```python
from build123d import *

# Parameters (mm, degrees)
SALIENTE_EXTRUIR1_DEPTH          = 3.1
SALIENTE_EXTRUIR2_DEPTH          = 3
SALIENTE_EXTRUIR3_DEPTH          = 3
TALADRO_DE_MARGEN_PARA_M41_D     = 4.5
TALADRO_DE_MARGEN_PARA_M41_DEPTH = 8.2
TALADRO_DE_MARGEN_PARA_M41_TIP   = 1.351936393
CROQUIS10_W                      = 11.5
CROQUIS10_H                      = 11.5
SALIENTE_EXTRUIR4_DEPTH          = 87
SALIENTE_EXTRUIR5_DEPTH          = 12
CROQUIS14_R                      = 2
CORTAR_EXTRUIR1_DEPTH            = 6
CHAFL_N1_SIZE                    = 0.3
TALADRO_DE_MARGEN_PARA_M61_D     = 6.6
TALADRO_DE_MARGEN_PARA_M61_DEPTH = 8.2
TALADRO_DE_MARGEN_PARA_M61_TIP   = 1.982840043
CORTAR_EXTRUIR3_DEPTH            = 12
REDONDEO1_R                      = 2.5
CROQUIS19_R                      = 6.15
SALIENTE_EXTRUIR6_DEPTH          = 12
CROQUIS20_R                      = 2.85
CORTAR_EXTRUIR4_DEPTH            = 8.2
CHAFL_N2_SIZE                    = 0.5


with BuildPart() as part:
    # Croquis4 → Saliente-Extruir1 (new body)
    with BuildSketch(Plane(origin=(0, 0, 6.1), x_dir=(-1, 0, 0), z_dir=(0, 0, -1))):
        with BuildLine():
            Line((-120.1, -80.5), (-120.1, 80.5))
            ThreePointArc((-120.1, 80.5), (-121.271572875, 83.328427125), (-124.1, 84.5))
            Line((-124.1, 84.5), (-329.1, 84.5))
            ThreePointArc((-329.1, 84.5), (-331.928427125, 83.328427125), (-333.1, 80.5))
            Line((-333.1, 80.5), (-333.1, -80.5))
            ThreePointArc((-333.1, -80.5), (-331.928427125, -83.328427125), (-329.1, -84.5))
            Line((-329.1, -84.5), (-124.1, -84.5))
            ThreePointArc((-124.1, -84.5), (-121.271572875, -83.328427125), (-120.1, -80.5))
        make_face()
    extrude(amount=SALIENTE_EXTRUIR1_DEPTH)



with BuildPart() as body_2:
    # Croquis5 → Saliente-Extruir2 (new body)
    with BuildSketch(Plane(origin=(0, 0, 3), x_dir=(-1, 0, 0), z_dir=(0, 0, -1))):
        with BuildLine():
            Line((-326.1, 59), (-326.1, -59))
            Line((-326.1, -59), (-326.1, -75))
            ThreePointArc((-326.1, -75), (-325.367766953, -76.767766953), (-323.6, -77.5))
            Line((-323.6, -77.5), (-129.6, -77.5))
            ThreePointArc((-129.6, -77.5), (-127.832233047, -76.767766953), (-127.1, -75))
            Line((-127.1, -75), (-127.1, 75))
            ThreePointArc((-127.1, 75), (-127.832233047, 76.767766953), (-129.6, 77.5))
            Line((-129.6, 77.5), (-323.6, 77.5))
            ThreePointArc((-323.6, 77.5), (-325.367766953, 76.767766953), (-326.1, 75))
            Line((-326.1, 75), (-326.1, 59))
        make_face()
        with BuildLine():
            Line((-324.1, 59), (-324.1, -59))
            Line((-324.1, -59), (-324.1, -75))
            ThreePointArc((-324.1, -75), (-323.953553391, -75.353553391), (-323.6, -75.5))
            Line((-323.6, -75.5), (-129.6, -75.5))
            ThreePointArc((-129.6, -75.5), (-129.246446609, -75.353553391), (-129.1, -75))
            Line((-129.1, -75), (-129.1, 75))
            ThreePointArc((-129.1, 75), (-129.246446609, 75.353553391), (-129.6, 75.5))
            Line((-129.6, 75.5), (-323.6, 75.5))
            ThreePointArc((-323.6, 75.5), (-323.953553391, 75.353553391), (-324.1, 75))
            Line((-324.1, 75), (-324.1, 59))
        make_face(mode=Mode.SUBTRACT)
    extrude(amount=SALIENTE_EXTRUIR2_DEPTH)


with BuildPart() as part_1:
    add(part.part)

    add(body_2.part)  # Saliente-Extruir3 merges body 2
    # Croquis6 → Saliente-Extruir3 (add)
    with BuildSketch(Plane(origin=(0, 0, 3), x_dir=(-1, 0, 0), z_dir=(0, 0, -1))):
        with BuildLine():
            Line((-120.1, -80.5), (-120.1, 80.5))
            ThreePointArc((-120.1, 80.5), (-121.271572875, 83.328427125), (-124.1, 84.5))
            Line((-124.1, 84.5), (-329.1, 84.5))
            ThreePointArc((-329.1, 84.5), (-331.928427125, 83.328427125), (-333.1, 80.5))
            Line((-333.1, 80.5), (-333.1, -80.5))
            ThreePointArc((-333.1, -80.5), (-331.928427125, -83.328427125), (-329.1, -84.5))
            Line((-329.1, -84.5), (-124.1, -84.5))
            ThreePointArc((-124.1, -84.5), (-121.271572875, -83.328427125), (-120.1, -80.5))
        make_face()
        with BuildLine():
            Line((-122.1, -80.5), (-122.1, 80.5))
            ThreePointArc((-122.1, 80.5), (-122.685786438, 81.914213562), (-124.1, 82.5))
            Line((-124.1, 82.5), (-329.1, 82.5))
            ThreePointArc((-329.1, 82.5), (-330.514213562, 81.914213562), (-331.1, 80.5))
            Line((-331.1, 80.5), (-331.1, -80.5))
            ThreePointArc((-331.1, -80.5), (-330.514213562, -81.914213562), (-329.1, -82.5))
            Line((-329.1, -82.5), (-124.1, -82.5))
            ThreePointArc((-124.1, -82.5), (-122.685786438, -81.914213562), (-122.1, -80.5))
        make_face(mode=Mode.SUBTRACT)
    extrude(amount=SALIENTE_EXTRUIR3_DEPTH)

    # Taladro de margen para M41
    with Locations(Plane.XY.offset(6.1)):
        with Locations((151.35, 20.5), (206.45, 20.5), (206.45, -20.5), (151.35, -20.5)):
            Hole(TALADRO_DE_MARGEN_PARA_M41_D / 2, depth=TALADRO_DE_MARGEN_PARA_M41_DEPTH)
            with Locations((0, 0, -(TALADRO_DE_MARGEN_PARA_M41_DEPTH + TALADRO_DE_MARGEN_PARA_M41_TIP / 2))):  # 118° drill point
                Cone(0, TALADRO_DE_MARGEN_PARA_M41_D / 2, TALADRO_DE_MARGEN_PARA_M41_TIP, mode=Mode.SUBTRACT)

    # Croquis10 → Saliente-Extruir4 (add)
    with BuildSketch(Plane(origin=(0, 0, 3), x_dir=(-1, 0, 0), z_dir=(0, 0, -1))):
        with Locations((-132.85, 71.75)):
            Rectangle(CROQUIS10_W, CROQUIS10_H)
        with Locations((-132.85, -71.75)):
            Rectangle(CROQUIS10_W, CROQUIS10_H)
        with Locations((-320.35, -71.75)):
            Rectangle(CROQUIS10_W, CROQUIS10_H)
        with Locations((-320.35, 71.75)):
            Rectangle(CROQUIS10_W, CROQUIS10_H)
    extrude(amount=SALIENTE_EXTRUIR4_DEPTH)

    # Croquis13 → Saliente-Extruir5 (add)
    with BuildSketch(Plane(origin=(0, 0, 3), x_dir=(-1, 0, 0), z_dir=(0, 0, -1))):
        Polygon((-213.1, -55), (-323.1, -55), (-323.1, 55), (-213.1, 55), (-213.1, 21.5), (-209.1, 21.5), (-209.1, 59), (-326.1, 59), (-326.1, -59), (-209.1, -59), (-209.1, -21.5), (-213.1, -21.5), align=None)
    extrude(amount=SALIENTE_EXTRUIR5_DEPTH)

    # Croquis14 → Cortar-Extruir1 (cut)
    with BuildSketch(Plane(origin=(0, 0, -84), x_dir=(-1, 0, 0), z_dir=(0, 0, -1))):
        with Locations((-132.85, -71.75)):
            Circle(CROQUIS14_R)
        with Locations((-132.85, 71.75)):
            Circle(CROQUIS14_R)
        with Locations((-320.35, 71.75)):
            Circle(CROQUIS14_R)
        with Locations((-320.35, -71.75)):
            Circle(CROQUIS14_R)
    extrude(amount=-CORTAR_EXTRUIR1_DEPTH, mode=Mode.SUBTRACT)

    # Chaflán1
    chafl_n1_edges = [part_1.edges().sort_by_distance(p)[0] for p in [
        (322.35, -71.75, -84),
        (322.35, 71.75, -84),
        (134.85, 71.75, -84),
        (134.85, -71.75, -84),
    ]]
    chamfer(chafl_n1_edges, length=CHAFL_N1_SIZE)

    # Taladro de margen para M61
    with Locations(Plane.XY.offset(6.1)):
        with Locations((229.4, 69.675), (229.4, -69.675)):
            Hole(TALADRO_DE_MARGEN_PARA_M61_D / 2, depth=TALADRO_DE_MARGEN_PARA_M61_DEPTH)
            with Locations((0, 0, -(TALADRO_DE_MARGEN_PARA_M61_DEPTH + TALADRO_DE_MARGEN_PARA_M61_TIP / 2))):  # 118° drill point
                Cone(0, TALADRO_DE_MARGEN_PARA_M61_D / 2, TALADRO_DE_MARGEN_PARA_M61_TIP, mode=Mode.SUBTRACT)

    # Croquis18 → Cortar-Extruir3 (cut)
    with BuildSketch(Plane(origin=(0, 0, -9), x_dir=(-1, 0, 0), z_dir=(0, 0, -1))):
        Polygon((-212.6, 21.5), (-212.6, 55.5), (-323.6, 55.5), (-323.6, -55.5), (-212.6, -55.5), (-212.6, -21.5), (-213.1, -21.5), (-213.1, -55), (-323.1, -55), (-323.1, 55), (-213.1, 55), (-213.1, 21.5), align=None)
    extrude(amount=-CORTAR_EXTRUIR3_DEPTH, mode=Mode.SUBTRACT)

    # Redondeo1
    redondeo1_edges = [part_1.edges().sort_by_distance(p)[0] for p in [
        (127.1, 77.5, -40.5),
        (127.1, -77.5, -40.5),
        (326.1, -77.5, -40.5),
        (326.1, 77.5, -40.5),
    ]]
    fillet(redondeo1_edges, radius=REDONDEO1_R)

    # Croquis19 → Saliente-Extruir6 (add)
    with BuildSketch(Plane(origin=(0, 0, 3), x_dir=(-1, 0, 0), z_dir=(0, 0, -1))):
        with Locations(Location((-151.35, -20.5, 0), (0, 0, 270))):
            Circle(CROQUIS19_R)
        with Locations(Location((-151.35, 20.5, 0), (0, 0, 270))):
            Circle(CROQUIS19_R)
        with Locations((-206.45, 20.5)):
            Circle(CROQUIS19_R)
        with Locations((-206.45, -20.5)):
            Circle(CROQUIS19_R)
    extrude(amount=SALIENTE_EXTRUIR6_DEPTH)

    # Croquis20 → Cortar-Extruir4 (cut)
    with BuildSketch(Plane.XY.offset(6.1)):
        with Locations((151.35, -20.5)):
            Circle(CROQUIS20_R)
        with Locations((206.45, -20.5)):
            Circle(CROQUIS20_R)
        with Locations((206.45, 20.5)):
            Circle(CROQUIS20_R)
        with Locations((151.35, 20.5)):
            Circle(CROQUIS20_R)
    extrude(amount=-CORTAR_EXTRUIR4_DEPTH, mode=Mode.SUBTRACT)

    # Chaflán2
    chafl_n2_edges = [part_1.edges().sort_by_distance(p)[0] for p in [
        (148.5, 20.5, 6.1),
        (203.6, 20.5, 6.1),
        (203.6, -20.5, 6.1),
        (148.5, -20.5, 6.1),
    ]]
    chamfer(chafl_n2_edges, length=CHAFL_N2_SIZE)


solid = part_1.part
```
CAD build for the part. Positions are in the model's coordinates, mm. A direction names the side the tool comes from. Give positions to 0.01 mm unless a question says otherwise; leave off trailing zeros. Loops run counter-clockwise (first coordinate to the right, second up) from the corner with the lowest first, then second, coordinate; pieces in that order, holes last. Notation, with made-up numbers: (61, -31) - (110, -31) arc R17 ccw to (110, -9) - close; hole circle Ø5 at (47.25, 39). An arc over 180 degrees is marked (long way). Put each result on its own line as item: value.
Q1. Slice it at B-B (x = 166). Give the cut face in (y, z), plus the area to 3 significant figures.
Filled in:
outline: (-84.5, 0) - (-82.5, 0) - (-82.5, 3) - (-77.5, 3) - (-77.5, 0) - (-75.5, 0) - (-75.5, 3) - (75.5, 3) - (75.5, 0) - (77.5, 0) - (77.5, 3) - (82.5, 3) - (82.5, 0) - (84.5, 0) - (84.5, 6.1) - (-84.5, 6.1) - close
area: 548 mm²
Q2. Mould opens along Y. For faces 4 (the face through (267, 59, -3)), 5 (the face through (228, 1, 6.1)), 6 (the face through (228, -84.5, 3)), 7 (the face through (206, 21, -2.1)) say: pulls with the +Y half, pulls with the -Y half, needs draft (parallel to the pull), parting line crosses it, or undercut.
Filled in:
face 4: undercut
face 5: needs draft
face 6: pulls with the -Y half
face 7: undercut
Q3. Slice it at A-A (z = -33). Give the cut face in (x, y).
Filled in:
outline: (127.1, -75) arc R2.5 ccw to (129.6, -77.5) - (138.6, -77.5) - (138.6, -66) - (127.1, -66) - close; (127.1, 66) - (138.6, 66) - (138.6, 77.5) - (129.6, 77.5) arc R2.5 ccw to (127.1, 75) - close; (314.6, -77.5) - (323.6, -77.5) arc R2.5 ccw to (326.1, -75) - (326.1, -66) - (314.6, -66) - close; (314.6, 66) - (326.1, 66) - (326.1, 75) arc R2.5 ccw to (323.6, 77.5) - (314.6, 77.5) - close
Q4. Flat gauge pins, fed straight in: pin 1 (8 mm diameter, centred on y = 6.5, z = -9.5, fed in from +X); pin 2 (9 mm diameter, centred on x = 133, z = -62, fed in from -Y); pin 3 (3 mm diameter, centred on x = 206, y = 21, fed in from +Z); pin 4 (6 mm diameter, centred on y = 62, z = -53.5, fed in from -X). Where does each tip first touch, or does it go through?
Filled in:
pin 1: stops at x = 326.1
pin 2: stops at y = -77.5
pin 3: stops at z = -2.1
pin 4: passes through
Q5. Probe line 1 along Y through (x, z) = (320, -81); line 2 along Y through (x, z) = (229.4, 4.9) (3 decimals); line 3 along X through (y, z) = (-68, -30). List the from-to ranges inside material, lowest first.
Filled in:
line 1: y = -77.5 to -73.72, -69.78 to -66, 66 to 69.78, 73.72 to 77.5
line 2: y = -84.5 to -72.975, -66.375 to 66.375, 72.975 to 84.5
line 3: x = 127.1 to 138.6, 314.6 to 326.1
Q6. Tool access for faces 1 (the face through (226.35, -70.94, 4.53)), 2 (the face through (227, -77.5, 2)), 3 (the face through (151, 21, -2.1)): list every direction of +Z, -Z, +X, -X, +Y, -Y with a clear straight run to the whole face (end or side of a thin tool).
Filled in:
face 1: +Z, -Z
face 2: -Z
face 3: +Z
Q7. Slice it at C-C (y = 42.5). Give the cut face in (x, z).
Filled in:
outline: (120.1, 0) - (122.1, 0) - (122.1, 3) - (127.1, 3) - (127.1, 0) - (129.1, 0) - (129.1, 3) - (209.1, 3) - (209.1, -9) - (212.6, -9) - (212.6, 3) - (323.6, 3) - (323.6, -9) - (326.1, -9) - (326.1, 3) - (331.1, 3) - (331.1, 0) - (333.1, 0) - (333.1, 6.1) - (120.1, 6.1) - close
